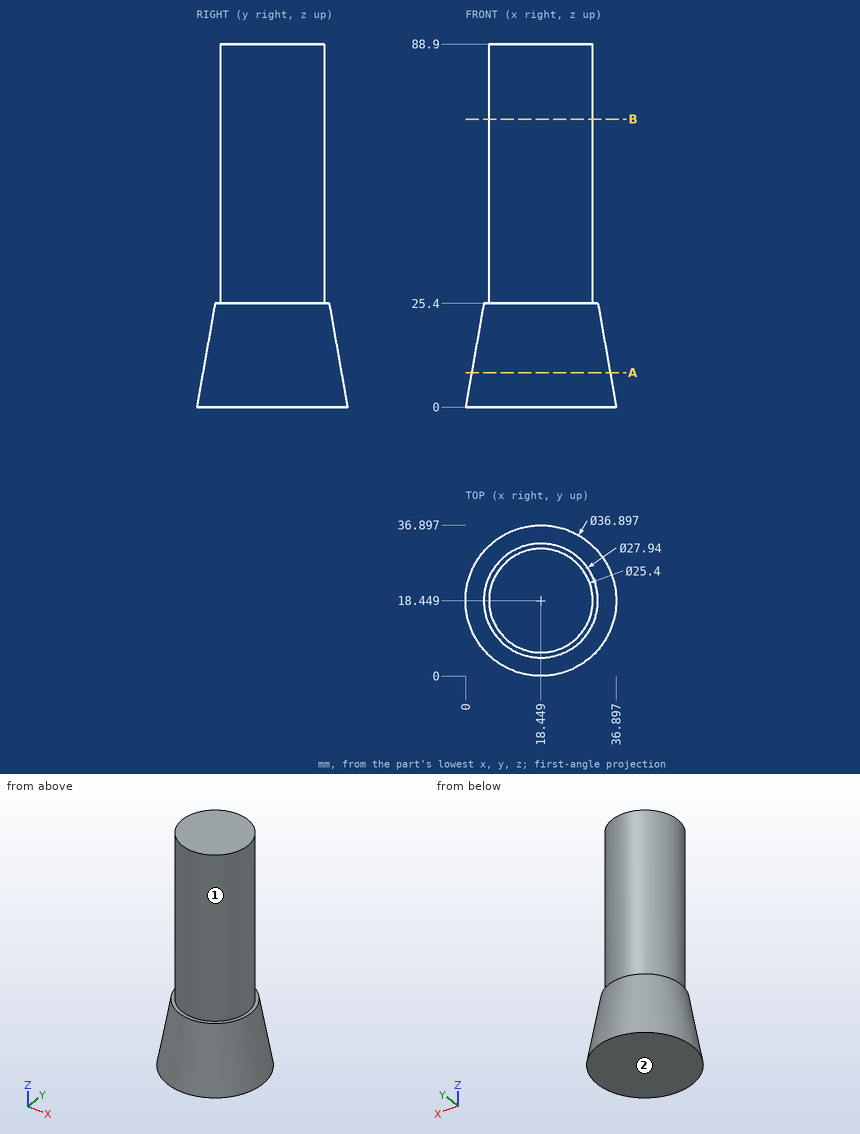
Could you check a few things on this drawing? It's one solid part, dimensions in mm from its lowest x, y, z. A direction names the side the tool comes from. Coordinates: 2 decimals unless noted, no trailing zeros. Loops run counter-clockwise (first coordinate to the right, second up) from the corner with the lowest first, then second, coordinate; pieces in that order, holes last. Notation, with made-up numbers: (80, 28) - (88, 28) arc R34 cw to (88, 66) - close; hole circle Ø1 at (-1, 89). An arc over 180 degrees is marked (long way). Return JSON: item names as keys, results as strings. Group by question number.
Item 1: If we section it at A-A on z = 8.5: Write out the boundary of the cut face in (x, y).
Item 2: Will these pins go through, and if not, where does the flat tip stop? P1, Ø10, axis at y = 17.5, z = 64, coming from the -X side; P2, Ø5, axis at y = 5, z = 59.5, coming from the -X side (1 decimal); P3, Ø2, axis at x = 33, z = 51, coming from the -Y side; P4, Ø8, axis at y = 16, z = 73, coming from the +X side.
Item 3: On a 3-axis mill with a long thin cutter (end or side, diameter ignored), from which of +Z, -Z, +X, -X, +Y, -Y can I reach the whole of each face in a straight line? I mean the marked faces 1 and 2. Say none if no direction works.
Item 4: I need wall thicknesses on line 1 (Z direction, x = 9, y = 9); line 2 (Y direction, x = 14, z = 12) (1 decimal); line 3 (Y direction, x = 23.5, z = 62.5) (1 decimal). Which ranges of each line are inside material? Lowest first, please. Write a range as from..to.
Item 5: If we section it at B-B on z = 70.5: Write out the boundary of the cut face in (x, y).
Calculated:
{
 "1": {"outline": "circle Ø33.9 at (18.45, 18.45)"},
 "2": {"P1": "stops at x = 5.75", "P2": "stops at x = 12", "P3": "passes through", "P4": "stops at x = 31.15"},
 "3": {"face 1": "+Z", "face 2": "-Z, +X, -X, +Y, -Y"},
 "4": {"line 1": "z = 0..25.4", "line 2": "y = 2.7..34.2", "line 3": "y = 6.8..30.1"},
 "5": {"outline": "circle Ø25.4 at (18.45, 18.45)"}
}
